Build history of the part. All positions in model axes, mm. Face numbers are marked on the shaded views. A direction names the side the tool comes from. Give positions to 0.01 mm unless a question says otherwise; leave off trailing zeros. Write each loop counter-clockwise with the first axis right and the second up, starting at its lowest first coordinate (ties: lowest second). Pieces come first, ordered by that corner, then holes. Notation, with made-up numbers: (61, 55) -> (117, 55) arc R22 cw to (117, 88) -> close; hole circle Ø5 at (45, 14.25). An arc over 180 degrees is marked (long way). One line per question, with ' | ' between items. Start each with the question number.
(1) Drill centre lines: probe 1 along Z at (x, y) = (74, -50); probe 2 along X at (y, z) = (-124, 8); probe 3 along Y at (x, z) = (-112, 17.5). Where is each one in solid material? Low to high. Write a range as from..to.
(2) Pin check, flat tips, straight feed: P1, Ø1.5, axis at x = -50.5, y = -101.5, coming from the +Z side; P2, Ø6, axis at y = -52.5, z = 40, coming from the +X side; P3, Ø12, axis at y = -19, z = 101.5, coming from the -X side; P4, Ø20.5, axis at x = 5, y = -56, coming from the +Z side. Stop position of each tip, or through.
(3) Band-saw the part on B-B, the plane y = -21. Give the cut face in (x, z), and give its area (3 significant figures).
(4) Band-saw the part on A-A, the plane z = 69. Give the cut face in (x, y), and give its area (3 significant figures).
(5) Band-saw the part on C-C, the plane z = -7. Give the cut face in (x, y).
(6) Band-saw the part on D-D, the plane x = -109.5. Give the cut face in (y, z).
(7) Tool access for the marked faces 5 and 6: list every direction of +Z, -Z, +X, -X, +Y, -Y with a clear straight run to the whole face (end or side of a thin tool).
(8) Pull direction Z, two halves, no side cores. Call the marked faces 1, 2, 3 and 4: released by +Z, released by -Z, zero draft, split by the parting line, or undercut.
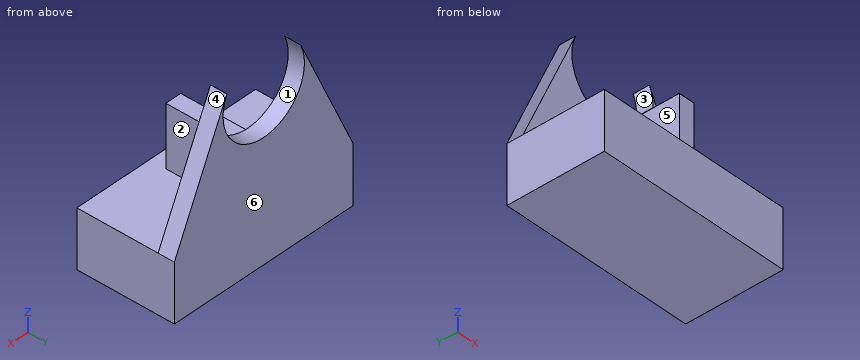
from build123d import *

# Parameters (mm, degrees)
F0_W     = 304.8
F0_H     = 89.688896
F1_DEPTH = 152.4
F2_DEPTH = 25.4
F4_DEPTH = 12.7


with BuildPart() as f1:
    # F0 (on Front) → F1 (new body)
    with BuildSketch(Plane.XZ):
        with Locations((-15.761086, -104.025281)):
            Rectangle(F0_W, F0_H)
    extrude(amount=F1_DEPTH)

    # F0 (on Front) → F2 (join)
    with BuildSketch(Plane.XZ):
        with BuildLine():
            Line((-78.707459, 134.241588), (-168.161086, -59.180833))
            Line((-168.161086, -59.180833), (136.638914, -59.180833))
            Line((136.638914, -59.180833), (47.185288, 134.241588))
            ThreePointArc((47.185288, 134.241588), (51.970658, 120.034148), (53.591021, 105.130271))
            ThreePointArc((53.591021, 105.130271), (-30.664962, 37.398527), (-78.707459, 134.241588))
        make_face()
    extrude(amount=F2_DEPTH)

    # F3 (on Right) → F4 (join, symmetric)
    with BuildSketch(Plane.YZ):
        Polygon((-23.240424, -61.891118), (-25.4, 35.778165), (-127, 35.778165), (-127, -61.891118), align=None)
    extrude(amount=F4_DEPTH, both=True)


solid = f1.part
Results:
1) probe 1: z = -148.87..-59.18 | probe 2: x = -12.7..12.7 | probe 3: y = -25.4..0
2) P1: stops at z = -59.18 | P2: passes through | P3: stops at x = -96.62 | P4: stops at z = 35.78
3) outline: (-168.16, -148.87) -> (136.64, -148.87) -> (136.64, -59.18) -> (47.19, 134.24) arc R69.35 cw to (53.59, 105.13) arc R69.35 cw (long way) to (-78.71, 134.24) -> (-168.16, -59.18) -> close | area: 57,500 mm²
4) outline: (-108.88, -25.4) -> (-74.96, -25.4) -> (-74.96, 0) -> (-108.88, 0) -> close; (43.44, -25.4) -> (77.36, -25.4) -> (77.36, 0) -> (43.44, 0) -> close | area: 1,720 mm²
5) outline: (-144.03, -25.4) -> (-12.7, -25.4) -> (-12.7, -127) -> (12.7, -127) -> (12.7, -25.4) -> (112.51, -25.4) -> (112.51, 0) -> (-144.03, 0) -> close
6) outline: (-152.4, -148.87) -> (0, -148.87) -> (0, 67.66) -> (-25.4, 67.66) -> (-25.4, -59.18) -> (-152.4, -59.18) -> close
7) face 5: +Z, -X, -Y | face 6: +Z, -Z, +X, -X, +Y
8) face 1: undercut | face 2: zero draft | face 3: undercut | face 4: released by +Z
